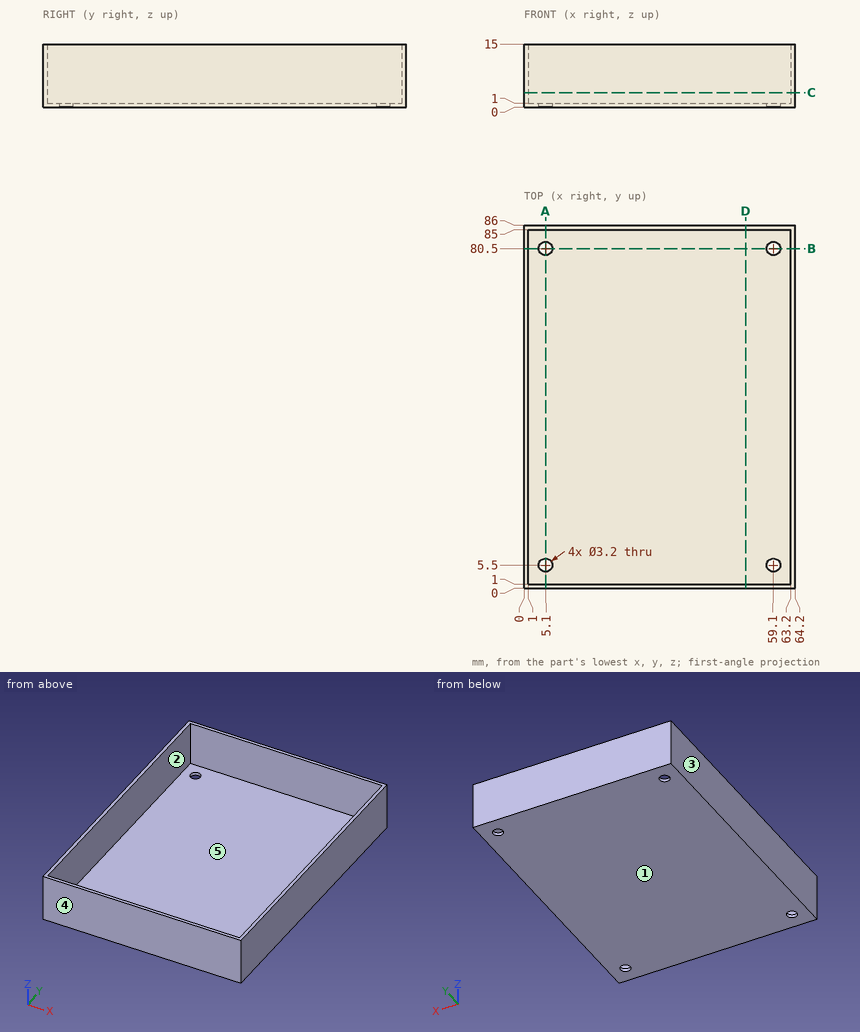
The drawing under review shows one solid part. Ordinate dimensions are in mm from its lowest x, y, z. A direction names the side the tool comes from. Give positions to 0.01 mm unless a question says otherwise; leave off trailing zeros. Order: outer loops, then holes, each group sorted by start corner. A loop starts at its lowest first (then second) coordinate and runs counter-clockwise, first axis right, second up. Notation, with made-up numbers: (59, 83) - (84, 83) arc R36 cw to (84, 121) - close; hole circle Ø9 at (63.25, -39). An arc over 180 degrees is marked (long way). Answer as a JSON object with one key per item and string values. Group by question number.
Item 1: Take a section at D-D on x = 52.5. Give the boundary of the cut face in (y, z).
Item 2: Draft analysis for pull direction X (two halves, no side actions). For the marked faces 3, 4 and 5, state which applies: pulls with the +X half, pulls with the -X half, needs draft (parallel to the pull), parting line crosses it, or undercut.
Item 3: Clearance check with flat-ended pins moving along their axes: pin 1 Ø10 at (x, y) = (26, 49) entering from -Z; pin 2 Ø4 at (x, y) = (59.1, 80.5) entering from +Z; pin 3 Ø3 at (x, y) = (59.1, 5.5) entering from +Z. State where each tip first meets the part, or that it passes through.
Item 4: Take a section at C-C on z = 3.5. Give the boundary of the cut face in (x, y), and give its area (3 significant figures).
Item 5: Take a section at A-A on x = 5.1. Give the boundary of the cut face in (y, z).
Item 6: Wall thickness on line 1 along Y through (x, z) = (59.1, 0.3); line 2 along X through (y, z) = (80.5, 0.25); line 3 along X through (y, z) = (80, 8.25): over which ranges is each line inside the solid? List them lowest first.
Item 7: Machinability: for the marked faces 1 and 2, which of the approach directions +Z, -Z, +X, -X, +Y, -Y give a long, thin tool a straight path to every point of the face, cutting with its end or side? Answer none if there is none.
Item 8: Take a section at B-B on y = 80.5. Give the boundary of the cut face in (x, z), and give its area (3 significant figures).
Reported:
{
 "1": {"outline": "(0, 0) - (86, 0) - (86, 15) - (85, 15) - (85, 1) - (1, 1) - (1, 15) - (0, 15) - close"},
 "2": {"face 3": "pulls with the -X half", "face 4": "needs draft", "face 5": "undercut"},
 "3": {"pin 1": "z = 0", "pin 2": "z = 1", "pin 3": "through"},
 "4": {"outline": "(0, 0) - (64.2, 0) - (64.2, 86) - (0, 86) - close; hole (1, 1) - (63.2, 1) - (63.2, 85) - (1, 85) - close", "area": "296 mm^2"},
 "5": {"outline": "(0, 0) - (3.9, 0) - (3.9, 1) - (1, 1) - (1, 15) - (0, 15) - close; (7.1, 0) - (78.9, 0) - (78.9, 1) - (7.1, 1) - close; (82.1, 0) - (86, 0) - (86, 15) - (85, 15) - (85, 1) - (82.1, 1) - close"},
 "6": {"line 1": "0 to 3.9, 7.1 to 78.9, 82.1 to 86", "line 2": "0 to 3.5, 6.7 to 57.5, 60.7 to 64.2", "line 3": "0 to 1, 63.2 to 64.2"},
 "7": {"face 1": "-Z, +X, -X, +Y, -Y", "face 2": "+Z"},
 "8": {"outline": "(0, 0) - (3.5, 0) - (3.5, 1) - (1, 1) - (1, 15) - (0, 15) - close; (6.7, 0) - (57.5, 0) - (57.5, 1) - (6.7, 1) - close; (60.7, 0) - (64.2, 0) - (64.2, 15) - (63.2, 15) - (63.2, 1) - (60.7, 1) - close", "area": "85.8 mm^2"}
}
